from build123d import *

# Parameters (mm, degrees)
F1_DEPTH = 24
F2_R     = 3
F3_DEPTH = 25
F4_START = -8
F4_DEPTH = 17
F5_DEPTH = 25
F6_DEPTH = 9
F7_DEPTH = 25
F8_R     = 2


with BuildPart() as f1:
    # F0 (on Top) → F1 (new body)
    with BuildSketch(Plane.XY):
        with BuildLine():
            ThreePointArc((3.7749172176, -4), (-5.5, 0), (3.7749172176, 4))
            Line((3.7749172176, 4), (18.7749172176, 4))
            Line((18.7749172176, 4), (18.7749172176, 8))
            Line((18.7749172176, 8), (18.7749172176, 12))
            Line((18.7749172176, 12), (3.7749172176, 12))
            Line((3.7749172176, 12), (-7.889866919, 12))
            Line((-7.889866919, 12), (-7.889866919, 4))
            ThreePointArc((-7.889866919, 4), (-6.3429648242, -6.1657762884), (3.7749172176, -8))
            Line((3.7749172176, -8), (18.7749172176, -8))
            Line((18.7749172176, -8), (18.7749172176, -4))
            Line((18.7749172176, -4), (3.7749172176, -4))
        make_face()
    extrude(amount=F1_DEPTH)

    # F2 (on Front) → F3 (cut, symmetric)
    with BuildSketch(Plane.XZ):
        with Locations((11.2749172176, 6)):
            Circle(F2_R)
        with Locations((11.2749172176, 18)):
            Circle(F2_R)
    extrude(amount=F3_DEPTH, both=True, mode=Mode.SUBTRACT)

    # F2 (on Front) → F4 (cut)
    with BuildSketch(Plane.XZ.offset(F4_START)):
        Polygon((13.7749172176, 13.6698729811), (16.2749172176, 18), (13.7749172176, 22.3301270189), (8.7749172176, 22.3301270189), (6.2749172176, 18), (8.7749172176, 13.6698729811), align=None)
        with Locations((11.2749172176, 18)):
            Circle(F2_R, mode=Mode.SUBTRACT)
        Polygon((8.7749172176, 10.3301270189), (6.2749172176, 6), (8.7749172176, 1.6698729811), (13.7749172176, 1.6698729811), (16.2749172176, 6), (13.7749172176, 10.3301270189), align=None)
        with Locations((11.2749172176, 6)):
            Circle(F2_R, mode=Mode.SUBTRACT)
    extrude(amount=-F4_DEPTH, mode=Mode.SUBTRACT)

    # F2 (on Front) → F5 (cut)
    with BuildSketch(Plane.XZ):
        with Locations((0, 12)):
            Circle(F2_R)
    extrude(amount=-F5_DEPTH, mode=Mode.SUBTRACT)

    # F2 (on Front) → F6 (cut)
    with BuildSketch(Plane.XZ):
        Polygon((2.5, 7.6698729811), (5, 12), (2.5, 16.3301270189), (-2.5, 16.3301270189), (-5, 12), (-2.5, 7.6698729811), align=None)
        with Locations((0, 12)):
            Circle(F2_R, mode=Mode.SUBTRACT)
        with Locations((0, 12)):
            Circle(F2_R)
        with BuildLine():
            ThreePointArc((2.5, 7.6698729811), (4.3301270189, 9.5), (5, 12))
            Line((5, 12), (2.5, 7.6698729811))
        make_face()
        with BuildLine():
            Line((2.5, 16.3301270189), (5, 12))
            ThreePointArc((5, 12), (4.3301270189, 14.5), (2.5, 16.3301270189))
        make_face()
        with BuildLine():
            Line((-2.5, 16.3301270189), (2.5, 16.3301270189))
            ThreePointArc((2.5, 16.3301270189), (0, 17), (-2.5, 16.3301270189))
        make_face()
        with BuildLine():
            Line((-5, 12), (-2.5, 16.3301270189))
            ThreePointArc((-2.5, 16.3301270189), (-4.3301270189, 14.5), (-5, 12))
        make_face()
        with BuildLine():
            ThreePointArc((-5, 12), (-4.3301270189, 9.5), (-2.5, 7.6698729811))
            Line((-2.5, 7.6698729811), (-5, 12))
        make_face()
        with BuildLine():
            ThreePointArc((-2.5, 7.6698729811), (0, 7), (2.5, 7.6698729811))
            Line((2.5, 7.6698729811), (-2.5, 7.6698729811))
        make_face()
    extrude(amount=-F6_DEPTH, mode=Mode.SUBTRACT)

    # F2 (on Front) → F7 (cut)
    with BuildSketch(Plane.XZ):
        with BuildLine():
            Line((-2.5, 16.3301270189), (2.5, 16.3301270189))
            ThreePointArc((2.5, 16.3301270189), (0, 17), (-2.5, 16.3301270189))
        make_face()
        Polygon((2.5, 7.6698729811), (5, 12), (2.5, 16.3301270189), (-2.5, 16.3301270189), (-5, 12), (-2.5, 7.6698729811), align=None)
        with Locations((0, 12)):
            Circle(F2_R, mode=Mode.SUBTRACT)
        with BuildLine():
            Line((2.5, 16.3301270189), (5, 12))
            ThreePointArc((5, 12), (4.3301270189, 14.5), (2.5, 16.3301270189))
        make_face()
        with BuildLine():
            ThreePointArc((2.5, 7.6698729811), (4.3301270189, 9.5), (5, 12))
            Line((5, 12), (2.5, 7.6698729811))
        make_face()
        with BuildLine():
            ThreePointArc((-2.5, 7.6698729811), (0, 7), (2.5, 7.6698729811))
            Line((2.5, 7.6698729811), (-2.5, 7.6698729811))
        make_face()
        with BuildLine():
            ThreePointArc((-5, 12), (-4.3301270189, 9.5), (-2.5, 7.6698729811))
            Line((-2.5, 7.6698729811), (-5, 12))
        make_face()
        with BuildLine():
            Line((-5, 12), (-2.5, 16.3301270189))
            ThreePointArc((-2.5, 16.3301270189), (-4.3301270189, 14.5), (-5, 12))
        make_face()
        with Locations((0, 12)):
            Circle(F2_R)
    extrude(amount=F7_DEPTH, mode=Mode.SUBTRACT)

    # F8
    f8_edges = [f1.edges().sort_by_distance(p)[0] for p in [
        (-7.889867, 12, 12),
        (-7.889867, 4, 12),
        (18.774917, -8, 12),
        (18.774917, 12, 12),
        (3.774917, -8, 19.63936),
        (3.774917, -8, 4.36064),
    ]]
    fillet(f8_edges, radius=F8_R)


solid = f1.part
Build history of the part. All positions in model axes, mm. A direction names the side the tool comes from. Coordinates: 2 decimals unless noted, no trailing zeros. Order: outer loops, then holes, each group sorted by start corner. A loop starts at its lowest first (then second) coordinate and runs counter-clockwise, first axis right, second up. Notation, with made-up numbers: (58.5, -13.75) - (89.5, -13.75) arc R19 ccw to (89.5, 23.25) - close; hole circle Ø5 at (-2.5, 78). An arc over 180 degrees is marked (long way). Write item = value, one per line. Start each with the question number.
1) Saw through at B-B on z = 20. Write the cut outline in (x, y).
2) Wall check: line 1 along Z through (x, y) = (11.25, 6); line 2 along Z through (x, y) = (13.5, 7.25); line 3 along Y through (x, z) = (7.5, 12.5). Give the ranges that are in metal, low to high. Write a range as from..to.
3) Two-plate mould, pull along X, no slides. Class faces 1 (the face through (12.66, 5.97, 3.34)), 2 (the face through (5, 6, 24)), 3 (the face through (-7.933, 4.038, 12.168)), 4 (the face through (12.66, -6.03, 15.34)): pulls with the +X half, pulls with the -X half, needs draft (parallel to the pull), parting line crosses it, or undercut.
4) Saw through at D-D on x = 13.25. Count the separate pieces of the cut face and the enclosed holes in it, then the cut area to 3 significant figures.
5) Saw through at A-A on x = 0. Write the cut outline in (y, z), then the cut area to 3 significant figures.
6) Saw through at C-C on x = -3.75. Write the cut outline in (y, z), then the cut area to 3 significant figures.
7) Flat gauge pins, fed straight in: pin 1 Ø5.5 at (x, z) = (11.27, 18) entering from -Y; pin 2 Ø12 at (x, z) = (12, 7) entering from -Y; pin 3 Ø1 at (y, z) = (2.5, 2.5) entering from -X; pin 4 Ø3 at (y, z) = (7, 15.5) entering from -X. Where does each tip first touch, or does it go through?
8) 3-axis set-ups, long thin cutter, end or side, ignore diameter. For faces 5 (the face through (10, -8, 12)), 6 (the face through (15.007, 9.972, 15.805)), 7 (the face through (11, 4, 12)): which of +Z, -Z, +X, -X, +Y, -Y reach the whole face in a straight line?
From the geometry:
q1.outline = (-8.07, 3.63) arc R8.85 ccw to (3.42, -8.16) arc R2 cw to (4.2, -8) - (9.04, -8) - (9.04, -4) - (3.77, -4) arc R5.5 cw (long way) to (3.77, 4) - (9.04, 4) - (9.04, 8) - (7.43, 8) - (7.43, 12) - (-5.89, 12) arc R2 ccw to (-7.89, 10) - (-7.89, 4.45) arc R2 cw to start; (13.51, -8) - (16.77, -8) arc R2 ccw to (18.77, -6) - (18.77, -4) - (13.51, -4) - close; (13.51, 4) - (18.77, 4) - (18.77, 10) arc R2 ccw to (16.77, 12) - (15.12, 12) - (15.12, 8) - (13.51, 8) - close
q2.line_1 = 0..3, 9..15, 21..24
q2.line_2 = 0..3.99, 8.01..15.99, 20.01..24
q2.line_3 = -8..-4, 4..12
q3.face_1 = undercut
q3.face_2 = needs draft
q3.face_3 = pulls with the -X half
q3.face_4 = undercut
q4.separate_pieces = 6
q4.enclosed_holes = 0
q4.area = 146 mm^2
q5.outline = (-8.85, 0) - (-5.5, 0) - (-5.5, 7) - (-8.85, 7) - close; (-8.85, 17) - (-5.5, 17) - (-5.5, 24) - (-8.85, 24) - close; (5.5, 0) - (12, 0) - (12, 9) - (9, 9) - (9, 7) - (5.5, 7) - close; (5.5, 17) - (9, 17) - (9, 15) - (12, 15) - (12, 24) - (5.5, 24) - close
q5.area = 150 mm^2
q6.outline = (-8.01, 0) - (-4.02, 0) - (-4.02, 8.69) - (-8.01, 8.69) - close; (-8.01, 15.31) - (-4.02, 15.31) - (-4.02, 24) - (-8.01, 24) - close; (4.02, 0) - (12, 0) - (12, 24) - (4.02, 24) - (4.02, 15.31) - (9, 15.31) - (9, 8.69) - (4.02, 8.69) - close
q6.area = 228 mm^2
q7.pin_1 = through
q7.pin_2 = -8
q7.pin_3 = -8.62
q7.pin_4 = -7.89
q8.face_5 = +Z, -Z, +X, -Y
q8.face_6 = +Y
q8.face_7 = +Z, -Z, +X
